Read the model definition and answer for the solid it produces. Units are mm, in the model's axes. Face numbers are marked on the shaded views. A direction names the side the tool comes from. Coordinates: 2 decimals unless noted, no trailing zeros. Write each loop counter-clockwise with the first axis right and the second up, starting at its lowest first coordinate (ties: lowest second). Pieces come first, ordered by that corner, then holes. Notation, with made-up numbers: (65, 25.25) -> (95, 25.25) arc R20 ccw to (95, 38.25) -> close; hole circle Ø7 at (-1, -15.75). An arc over 180 degrees is marked (long way). One line per item, written item: value. Start each with the question number.
1. Find section C-C, the plane z = 21.75. Write down the section's boundary in (x, y), and give its area (3 significant figures).
2. Given P1, Ø3, axis at x = -30.5, y = -48.5, coming from the +Z side; P2, Ø1, axis at x = -24.5, z = 20, coming from the -Y side; P3, Ø3, axis at x = -19.5, z = 22.5, coming from the -Y side, each flat-ended and moving along its own axis, determine where each tip first touches the part or whether it passes through.
3. For the marked faces 1, 2 and 3, determine the directions among +Z, -Z, +X, -X, +Y, -Y from which every point of the face is accessible in a straight line to the end or side of a thin tool.
4. Consider line 1 along Z through (x, y) = (-3, 17); line 2 along Y through (x, z) = (-12, 25.75); line 3 along Z through (x, y) = (1, 7.5). Determine where each line is inside the solid, lowest interval first.
5. Find section A-A, the plane x = -12. Write down the section's boundary in (y, z), and give its area (3 significant figures).
6. Find section B-B, the plane y = 27. Write down the section's boundary in (x, z), and give its area (3 significant figures).
```python
from build123d import *

# Parameters (mm, degrees)
PAD041_START        = 0.3
PAD041_DEPTH        = 41.4
HOLE006_D           = 2.6
HOLE006_DEPTH       = 3
HOLE006_CBORE_D     = 3.5
HOLE006_CBORE_DEPTH = 1
HOLE006_TIPS_R      = 1.3
POCKET012_DEPTH     = 3
HOLE007_D           = 2.6
HOLE007_DEPTH       = 4
HOLE007_CBORE_D     = 3.5
HOLE007_CBORE_DEPTH = 1


with BuildPart() as part:
    # Sketch063 (on Face1 of CopyPocket007) → Pad041 (new body)
    with BuildSketch(Plane.YZ.offset(-38.919239).offset(PAD041_START)):
        with BuildLine():
            Line((58.243801, 33.999995), (15.243801, 33.999995))
            ThreePointArc((15.243801, 33.999995), (6.279309, 32.328219), (-1.480028, 27.53764))
            Line((-1.480028, 27.53764), (-11.145172, 18.757006))
            ThreePointArc((-20.627205, 15.092996), (-15.54454, 16.040855), (-11.145172, 18.757006))
            Line((-20.627205, 15.092996), (-50.3848, 15.092996))
            Line((-50.3848, 15.092996), (-50.3848, 13.092994))
            Line((-20.627205, 13.092994), (-50.3848, 13.092994))
            ThreePointArc((-20.627205, 13.092994), (-15.54454, 14.040853), (-11.14517, 16.757003))
            Line((-1.480025, 25.537638), (-11.14517, 16.757003))
            ThreePointArc((15.243801, 31.999992), (6.27931, 30.328217), (-1.480025, 25.537638))
            Line((58.243801, 31.999992), (15.243801, 31.999992))
            Line((58.243801, 33.999995), (58.243801, 31.999992))
        make_face()
    extrude(amount=PAD041_DEPTH)

    # Hole006
    with Locations(Plane.XY.offset(33.999995)):
        with Locations((-36.423248, 19.105118), (0.57751, 43.077087), (-15.945976, 55.996437)):
            CounterBoreHole(HOLE006_D / 2, HOLE006_CBORE_D / 2, HOLE006_CBORE_DEPTH, depth=HOLE006_DEPTH)

    # Hole006 tips → Hole006 tip 1 section 0
    with BuildSketch(Plane.XY.offset(30.999995), mode=Mode.PRIVATE) as hole006_tip_1_s0:
        with Locations((-36.423248, 19.105118)):
            Circle(HOLE006_TIPS_R)
    loft([hole006_tip_1_s0.sketch, Vertex(-36.423248, 19.105118, 30.218876)], mode=Mode.SUBTRACT)

    # Hole006 tips → Hole006 tip 2 section 0
    with BuildSketch(Plane.XY.offset(30.999995), mode=Mode.PRIVATE) as hole006_tip_2_s0:
        with Locations((0.57751, 43.077087)):
            Circle(HOLE006_TIPS_R)
    loft([hole006_tip_2_s0.sketch, Vertex(0.57751, 43.077087, 30.218876)], mode=Mode.SUBTRACT)

    # Hole006 tips → Hole006 tip 3 section 0
    with BuildSketch(Plane.XY.offset(30.999995), mode=Mode.PRIVATE) as hole006_tip_3_s0:
        with Locations((-15.945976, 55.996437)):
            Circle(HOLE006_TIPS_R)
    loft([hole006_tip_3_s0.sketch, Vertex(-15.945976, 55.996437, 30.218876)], mode=Mode.SUBTRACT)

    # Sketch065 (on Face12 of Hole006) → Pocket012 (cut)
    with BuildSketch(Plane.XY.offset(15.092996)):
        with BuildLine():
            Line((-37.458851, -25.793337), (-37.458851, -37.953597))
            ThreePointArc((-37.458851, -37.953597), (-36.711973, -39.756719), (-34.908851, -40.503597))
            Line((-34.908851, -40.503597), (-24.089139, -40.503597))
            ThreePointArc((-24.089139, -40.503597), (-22.286017, -39.756719), (-21.539139, -37.953597))
            Line((-21.539139, -37.953597), (-21.539139, -25.793337))
            ThreePointArc((-21.539139, -25.793337), (-22.286017, -23.990215), (-24.089139, -23.243337))
            Line((-24.089139, -23.243337), (-34.908851, -23.243337))
            ThreePointArc((-34.908851, -23.243337), (-36.711973, -23.990215), (-37.458851, -25.793337))
        make_face()
    extrude(amount=-POCKET012_DEPTH, mode=Mode.SUBTRACT)

    # Hole007
    with Locations(Plane.XY.offset(15.092996)):
        with Locations((-4.888495, -47.913956), (-30.924999, -47.913956)):
            CounterBoreHole(HOLE007_D / 2, HOLE007_CBORE_D / 2, HOLE007_CBORE_DEPTH, depth=HOLE007_DEPTH)


solid = part.part
```
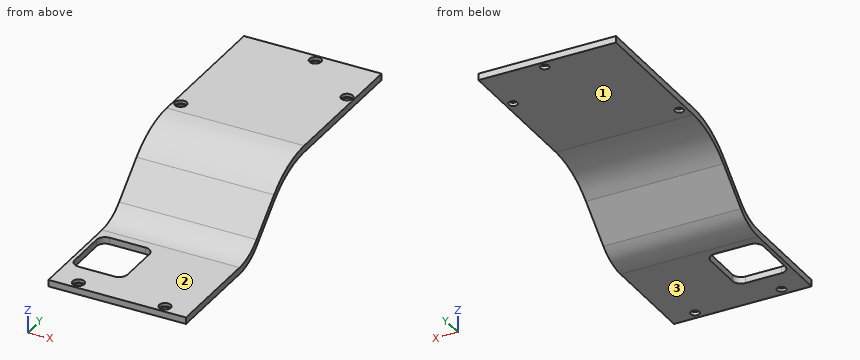
Answer block:
1. outline: (-38.62, -7.85) -> (2.78, -7.85) -> (2.78, -5.65) -> (-38.62, -5.65) -> close
1. area: 91.1 mm2
2. P1: stops at z = 15.09
2. P2: stops at y = -10.33
2. P3: stops at y = -8.68
3. face 1: -Z, +X, -X, +Y
3. face 2: +Z, +X, -X, -Y
3. face 3: -Z, +X, -X, +Y, -Y
4. line 1: z = 32 to 34
4. line 2: y = -3.45 to -1.24
4. line 3: z = 30.76 to 32.76
5. outline: (-50.38, 13.09) -> (-20.63, 13.09) arc R14.1 ccw to (-11.15, 16.76) -> (-1.48, 25.54) arc R24.87 cw to (15.24, 32) -> (58.24, 32) -> (58.24, 34) -> (15.24, 34) arc R24.87 ccw to (-1.48, 27.54) -> (-11.15, 18.76) arc R14.1 cw to (-20.63, 15.09) -> (-50.38, 15.09) -> close
5. area: 217 mm2
6. outline: (-38.62, 32) -> (2.78, 32) -> (2.78, 34) -> (-38.62, 34) -> close
6. area: 82.8 mm2
